```python
from build123d import *

# Parameters (mm, degrees)
SKETCH1_W           = 52.000002935
SKETCH1_H           = 18.000001088
SKETCH1_R           = 1.599502817
BOSS_EXTRUDE1_DEPTH = 2.999998629
SKETCH2_W           = 4
SKETCH2_H           = 30
CUT_EXTRUDE1_DEPTH  = 84.68851942
FILLET1_R           = 5


with BuildPart() as part:
    # Sketch1 → Boss-Extrude1 (new body)
    with BuildSketch(Plane(origin=(120.988696814, 0, 0), x_dir=(0, -1, 0), z_dir=(-1, 0, 0))):
        with Locations((49.005120062, 27.999999933)):
            Rectangle(SKETCH1_W, SKETCH1_H)
        with Locations(Location((26.005118371, 32.999999236, 0), (0, 0, 90))):
            Circle(SKETCH1_R, mode=Mode.SUBTRACT)
        with Locations(Location((26.005118371, 23.000000115, 0), (0, 0, 90))):
            Circle(SKETCH1_R, mode=Mode.SUBTRACT)
        with Locations(Location((72.005118202, 32.999999236, 0), (0, 0, 90))):
            Circle(SKETCH1_R, mode=Mode.SUBTRACT)
        with Locations(Location((72.005118202, 23.000000115, 0), (0, 0, 90))):
            Circle(SKETCH1_R, mode=Mode.SUBTRACT)
    extrude(amount=-BOSS_EXTRUDE1_DEPTH)

    # Sketch2 → Cut-Extrude1 (cut, through all)
    with BuildSketch(Plane.ZY.offset(-120.988696814)):
        with Locations((35.000000477, -49.005120061)):
            Rectangle(SKETCH2_W, SKETCH2_H)
        Polygon((33.000000477, -34.005120061), (37.000000477, -34.005120061), (37.000000477, -30.005120061), align=None)
        Polygon((22.999999389, -34.005120061), (18.999999389, -30.005120061), (18.999999389, -34.005120061), align=None)
        with Locations((20.999999389, -49.005120061)):
            Rectangle(SKETCH2_W, SKETCH2_H)
        Polygon((22.999999389, -64.005120061), (18.999999389, -64.005120061), (18.999999389, -68.005120061), align=None)
        Polygon((37.000000477, -68.005120061), (37.000000477, -64.005120061), (33.000000477, -64.005120061), align=None)
    extrude(amount=-CUT_EXTRUDE1_DEPTH, mode=Mode.SUBTRACT)

    # Fillet1
    fillet1_edges = [part.edges().sort_by_distance(p)[0] for p in [
        (122.488696128, -34.005120061, 22.999999389),
        (122.488696128, -64.005120061, 22.999999389),
        (122.488696128, -64.005120061, 33.000000477),
        (122.488696128, -34.005120061, 33.000000477),
    ]]
    fillet(fillet1_edges, radius=FILLET1_R)


solid = part.part
```
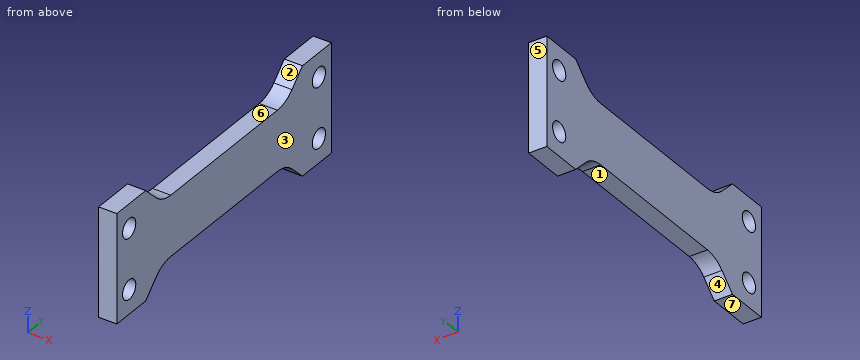
CAD build for the part. Positions are in the model's coordinates, mm. Face numbers are marked on the shaded views. A direction names the side the tool comes from. Round coordinates to 2 decimals unless told otherwise and drop trailing zeros. Order: outer loops, then holes, each group sorted by start corner. A loop starts at its lowest first (then second) coordinate and runs counter-clockwise, first axis right, second up. Notation, with made-up numbers: (-36.5, 83.25) - (-12.5, 83.25) arc R34 ccw to (-12.5, 116.25) - close; hole circle Ø4 at (9, 5.5). An arc over 180 degrees is marked (long way). Use CSV: the item, a comma, the result in double quotes. Start each with the question number.
1) Two-plate mould, pull along Y, no slides. Class the marked faces 4, 5, 6 and 7: pulls with the +Y half, pulls with the -Y half, needs draft (parallel to the pull), parting line crosses it, or undercut.
2) Saw through at B-B (x = 123.45). List the corners of the cut face in (y, z).
3) Tool access for the marked faces 1, 2 and 3: list every direction of +Z, -Z, +X, -X, +Y, -Y with a clear straight run to the whole face (end or side of a thin tool).
4) Saw through at C-C (y = -58). List the corners of the cut face in (x, z), and give its area (3 significant figures).
5) Saw through at A-A (z = 34). List the corners of the cut face in (x, y).
6) Saw through at D-D (z = 22.25). List the corners of the cut face in (x, y), and give its area (3 significant figures).
7) Wall check: L1, parallel to Y at x = 123.7, z = 20; L2, parallel to Z at x = 122.25, y = -54; L3, parallel to Y at x = 122.7, z = 20.75. Give the ranges that are in metal, low to high. Write a range as [from, to].
8) Pin check, flat tips, straight feed: pin 1 Ø2.5 at (y, z) = (-26.01, 23) entering from +X; pin 2 Ø0.9 at (x, y) = (123, -51) entering from -Z. Stop position of each tip, or through.
Values follow:
1,face 4,"undercut"
1,face 5,"pulls with the +Y half"
1,face 6,"undercut"
1,face 7,"needs draft"
2,outline,"(-75.01, 19) - (-68.01, 19) - (-65.47, 21.54) arc R5 cw to (-61.93, 23) - (-36.08, 23) arc R5 cw to (-32.54, 21.54) - (-30.01, 19) - (-23.01, 19) - (-23.01, 37) - (-30.01, 37) - (-32.54, 34.46) arc R5 cw to (-36.08, 33) - (-61.93, 33) arc R5 cw to (-65.47, 34.46) - (-68.01, 37) - (-75.01, 37) - close; hole circle Ø3.2 at (-72.01, 23); hole circle Ø3.2 at (-72.01, 33); hole circle Ø3.2 at (-26.01, 23); hole circle Ø3.2 at (-26.01, 33)"
3,face 1,"-Z, +X, -X"
3,face 2,"+Z, +X, -X"
3,face 3,"+Z, -Z, +X, +Y, -Y"
4,outline,"(120.99, 23) - (123.99, 23) - (123.99, 33) - (120.99, 33) - close"
4,area,"30.0 mm2"
5,outline,"(120.99, -75.01) - (123.99, -75.01) - (123.99, -73.25) - (120.99, -73.25) - close; (120.99, -70.76) - (123.99, -70.76) - (123.99, -64.93) - (120.99, -64.93) - close; (120.99, -33.08) - (123.99, -33.08) - (123.99, -27.25) - (120.99, -27.25) - close; (120.99, -24.76) - (123.99, -24.76) - (123.99, -23.01) - (120.99, -23.01) - close"
6,outline,"(120.99, -75.01) - (123.99, -75.01) - (123.99, -73.42) - (120.99, -73.42) - close; (120.99, -70.59) - (123.99, -70.59) - (123.99, -64.57) - (120.99, -64.57) - close; (120.99, -33.44) - (123.99, -33.44) - (123.99, -27.42) - (120.99, -27.42) - close; (120.99, -24.59) - (123.99, -24.59) - (123.99, -23.01) - (120.99, -23.01) - close"
6,area,"45.7 mm2"
7,L1,"y = [-75.01, -67.01], [-31.01, -23.01]"
7,L2,"z = [23, 33]"
7,L3,"y = [-75.01, -66.26], [-31.76, -23.01]"
8,pin 1,"passes through"
8,pin 2,"stops at z = 23"
